from build123d import *

# Parameters (mm, degrees)
F1_DEPTH = 304.8


with BuildPart() as f1:
    # F0 (on Front) → F1 (new body)
    with BuildSketch(Plane.XZ):
        with BuildLine():
            Line((0, 50.8), (0, 0))
            Line((0, 0), (2.40839, 0))
            ThreePointArc((2.40839, 0), (3.99589, 0.425369), (5.158021, 1.5875))
            Line((5.158021, 1.5875), (15.24, 19.05))
            Line((15.24, 19.05), (26.796055, 50.8))
            Line((26.796055, 50.8), (0, 50.8))
        make_face()
    extrude(amount=F1_DEPTH)

    # F2: F1 across face


with BuildPart() as f1_1:
    add(f1.part)
    add(f1.part.mirror(Plane(origin=(0, -152.4, 25.4), x_dir=(0, -1, 0), z_dir=(-1, 0, 0))))


solid = f1_1.part
The listing builds one solid part. Answer for the finished solid, in the listing's coordinates (mm). Give positions to 0.01 mm unless a question says otherwise; leave off trailing zeros. Loops run counter-clockwise (first coordinate to the right, second up) from the corner with the lowest first, then second, coordinate; pieces in that order, holes last. Notation, with made-up numbers: M 60,12 L 101,12 A28 ccw 101,32 Z; hole C -7.75,-33.5 d11. An arc over 180 degrees is marked long. Answer as CSV lines item,"result".
Item 1: Straight lines are drawn through the part: line 1 along X through (y, z) = (-128.5, 28); line 2 along X through (y, z) = (-129.5, 24.5); line 3 along Z through (x, y) = (9, -91.5). For each, find the intervals that lie inside material, in ascending order. Write a range as [from, to].
Values follow:
line 1,"x = [-18.5, 18.5]"
line 2,"x = [-17.22, 17.22]"
line 3,"z = [8.24, 50.8]"
Item 2: Given pin 1 Ø4 at (x, z) = (-13.5, 9.5) entering from +Y; pin 2 Ø10 at (y, z) = (-101, 18) entering from -X; pin 3 Ø1 at (x, y) = (-13.5, -179.5) entering from -Z; pin 4 Ø1 at (y, z) = (-80.5, 26) entering from +X, each flat-ended and moving along its own axis, determine where each tip first touches the part or whether it passes through.
Values follow:
pin 1,"passes through"
pin 2,"stops at x = -16.68"
pin 3,"stops at z = 15.17"
pin 4,"stops at x = 17.95"
Item 3: The part is cut by section B-B (x = -20). Give the vertices of the cut face in (y, z), and give its area (3 significant figures).
Values follow:
outline,"M -304.8,32.13 L 0,32.13 L 0,50.8 L -304.8,50.8 Z"
area,"5,690 mm^2"
Item 4: The part is cut by section C-C (z = 5). Give the vertices of the cut face in (x, y), and give its area (3 significant figures).
Values follow:
outline,"M -7.13,-304.8 L 7.13,-304.8 L 7.13,0 L -7.13,0 Z"
area,"4,350 mm^2"
